The figure shows three views and two pictorial views of one solid part (mm, origin at its lowest corner). Answer the questions. Coordinates: 2 decimals unless noted, no trailing zeros. Order: outer loops, then holes, each group sorted by start corner. A loop starts at its lowest first (then second) coordinate and runs counter-clockwise, first axis right, second up. Notation, with made-up numbers: (30, 87) -> (35, 87) arc R11 cw to (35, 101) -> close; hole circle Ø3 at (83.25, -34.5). An arc over 180 degrees is marked (long way). Return JSON: item names as keys, results as strings.
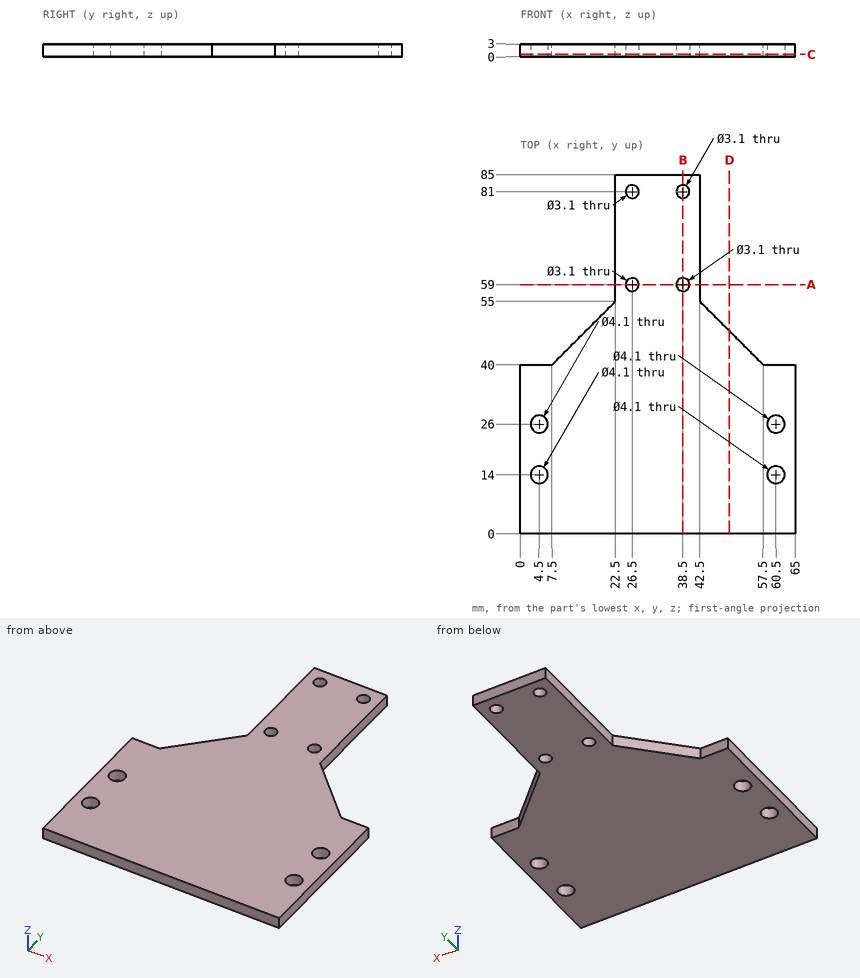
1. Each of these flat-tipped pins is pushed along its axis until it touches: pin 1 Ø0.9 at (x, z) = (63, 1.5) entering from +Y; pin 2 Ø3.5 at (x, y) = (4.5, 14) entering from -Z; pin 3 Ø1 at (y, z) = (58, 2) entering from -X; pin 4 Ø1.5 at (y, z) = (52.5, 1.5) entering from -X. Where does it stop, or does it pass through?
Answer block:
{"pin 1": "stops at y = 40", "pin 2": "passes through", "pin 3": "stops at x = 22.5", "pin 4": "stops at x = 19.25"}
2. The part is cut by section C-C on z = 0.55. Give the number of separate pieces and of enclosed holes in the cut face, and give its area (3 significant figures).
Answer block:
{"separate pieces": "1", "enclosed holes": "8", "area": "3,640 mm2"}
3. The part is cut by section A-A on y = 59. Give the vertices of the cut face in (x, z), and give its area (3 significant figures).
Answer block:
{"outline": "(22.5, 0) -> (24.95, 0) -> (24.95, 3) -> (22.5, 3) -> close; (28.05, 0) -> (36.95, 0) -> (36.95, 3) -> (28.05, 3) -> close; (40.05, 0) -> (42.5, 0) -> (42.5, 3) -> (40.05, 3) -> close", "area": "41.4 mm2"}
4. The part is cut by section B-B on x = 38.5. Give the vertices of the cut face in (y, z), and give its area (3 significant figures).
Answer block:
{"outline": "(0, 0) -> (57.45, 0) -> (57.45, 3) -> (0, 3) -> close; (60.55, 0) -> (79.45, 0) -> (79.45, 3) -> (60.55, 3) -> close; (82.55, 0) -> (85, 0) -> (85, 3) -> (82.55, 3) -> close", "area": "236 mm2"}
5. Consider line 1 (Y direction, x = 26.5, z = 1.95); line 2 (X direction, y = 27, z = 1.3); line 3 (X direction, y = 76, z = 2). Determine where each line is inside the solid, lowest interval first. Write a range as from..to.
Answer block:
{"line 1": "y = 0..57.45, 60.55..79.45, 82.55..85", "line 2": "x = 0..2.71, 6.29..58.71, 62.29..65", "line 3": "x = 22.5..42.5"}
6. The part is cut by section D-D on x = 49.5. Give the vertices of the cut face in (y, z).
Answer block:
{"outline": "(0, 0) -> (48, 0) -> (48, 3) -> (0, 3) -> close"}
